```python
from build123d import *

# Parameters (mm, degrees)
F0_W      = 300
F0_H      = 160
F1_DEPTH  = 10
F2_R      = 25
F3_DEPTH  = 20.001
F4_R      = 5.5
F5_DEPTH  = 10
F6_W      = 300
F6_H      = 15
F7_DEPTH  = 20.001
F8_R      = 20
F9_R      = 27.5
F10_DEPTH = 13


with BuildPart() as f1:
    # F0 (on Front) → F1 (new body, symmetric)
    with BuildSketch(Plane.XZ):
        Rectangle(F0_W, F0_H)
    extrude(amount=F1_DEPTH, both=True)

    # F2 (on face) → F3 (cut, through all)
    with BuildSketch(Plane.XZ.offset(10)):
        with Locations((-75, 0)):
            Circle(F2_R)
        with Locations((75, 0)):
            Circle(F2_R)
    extrude(amount=-F3_DEPTH, mode=Mode.SUBTRACT)

    # F4 (on face) → F5 (cut)
    with BuildSketch(Plane.XZ.offset(10)):
        with Locations((-137.5, 0)):
            Circle(F4_R)
        with Locations((0, 50)):
            Circle(F4_R)
        with Locations((137.5, 0)):
            Circle(F4_R)
        with Locations((0, -50)):
            Circle(F4_R)
    extrude(amount=-F5_DEPTH, mode=Mode.SUBTRACT)

    # F6 (on face) → F7 (cut, through all)
    with BuildSketch(Plane.XZ.offset(10)):
        with Locations((0, -72.5)):
            Rectangle(F6_W, F6_H)
    extrude(amount=-F7_DEPTH, mode=Mode.SUBTRACT)

    # F8
    f8_edges = [f1.edges().sort_by_distance(p)[0] for p in [
        (-150, 0, 80),
        (150, 0, 80),
        (-150, 0, -65),
        (150, 0, -65),
    ]]
    fillet(f8_edges, radius=F8_R)

    # F9 (on face) → F10 (cut)
    with BuildSketch(Plane.XZ.offset(10)):
        with Locations((-75, 0)):
            Circle(F9_R)
        with Locations((75, 0)):
            Circle(F9_R)
    extrude(amount=-F10_DEPTH, mode=Mode.SUBTRACT)


solid = f1.part
```
The model under review builds one solid part; all positions refer to its coordinate system, in mm. A direction names the side the tool comes from. Round coordinates to 2 decimals unless told otherwise and drop trailing zeros. Loops run counter-clockwise (first coordinate to the right, second up) from the corner with the lowest first, then second, coordinate; pieces in that order, holes last. Notation, with made-up numbers: (33, 79) - (88, 79) arc R30 cw to (88, 102) - close; hole circle Ø4 at (-27, -18.75). An arc over 180 degrees is marked (long way). Write each question's results on one line, items separated by ' | '. Start each with the question number.
Q1. Take a section at C-C on y = 6. Give the boundary of the cut face in (x, z), plus the area to 3 significant figures.
Q2. Wall thickness on line 1 along Z through (x, y) = (0, -6.75); line 2 along X through (y, z) = (-9, -25); line 3 along Z through (x, y) = (-75, 0): over which ranges is each line inside the solid? List them lowest first. Write a range as [from, to].
Q3. Take a section at B-B on x = 75. Give the boundary of the cut face in (y, z).
Q4. Draft analysis for pull direction X (two halves, no side actions). For faces 3 (the cylindrical face through (143.986, 0.14, 74.297)), 4 (the cylindrical face through (-144.297, 0.14, -58.986)), 5 (the cylindrical face through (47.527, -3.591, 1.209)), 6 (the flat face through (-2, 0, -65)), state which applies: pulls with the +X half, pulls with the -X half, needs draft (parallel to the pull), parting line crosses it, or undercut.
Q5. Take a section at D-D on z = 50. Give the boundary of the cut face in (x, y).
Q6. Insertion check: P1, Ø5.5, axis at x = 139.5, z = 2.5, coming from the -Y side; P2, Ø10, axis at x = 0, z = 50, coming from the -Y side. Each pin has a flat end and moves straight along its axis. Give the tip position at first contact, or say it passes through.
Q7. Take a section at A-A on z = 0. Give the boundary of the cut face in (x, y), plus the area to 3 significant figures.
Q8. Tool access review of faces 1 (the cylindrical face through (-102.473, -3.591, 1.209)), 2 (the flat face through (-2, -10, 9)): name each direction out of +Z, -Z, +X, -X, +Y, -Y from which nothing blocks a thin tool from reaching the whole face with its end or side.
Data:
1) outline: (-150, -45) arc R20 ccw to (-130, -65) - (130, -65) arc R20 ccw to (150, -45) - (150, 60) arc R20 ccw to (130, 80) - (-130, 80) arc R20 ccw to (-150, 60) - close; hole circle Ø50 at (-75, 0); hole circle Ø50 at (75, 0) | area: 39,200 mm²
2) line 1: z = [-65, -55.5], [-44.5, 44.5], [55.5, 80] | line 2: x = [-150, -86.46], [-63.54, 63.54], [86.46, 150] | line 3: z = [-65, -27.5], [27.5, 80]
3) outline: (-10, -65) - (10, -65) - (10, -25) - (3, -25) - (3, -27.5) - (-10, -27.5) - close; (-10, 27.5) - (3, 27.5) - (3, 25) - (10, 25) - (10, 80) - (-10, 80) - close
4) face 3: pulls with the +X half | face 4: pulls with the -X half | face 5: undercut | face 6: needs draft
5) outline: (-150, -10) - (-5.5, -10) - (-5.5, 0) - (5.5, 0) - (5.5, -10) - (150, -10) - (150, 10) - (-150, 10) - close
6) P1: stops at y = -10 | P2: stops at y = 0
7) outline: (-150, -10) - (-143, -10) - (-143, 0) - (-132, 0) - (-132, -10) - (-102.5, -10) - (-102.5, 3) - (-100, 3) - (-100, 10) - (-150, 10) - close; (-50, 3) - (-47.5, 3) - (-47.5, -10) - (47.5, -10) - (47.5, 3) - (50, 3) - (50, 10) - (-50, 10) - close; (100, 3) - (102.5, 3) - (102.5, -10) - (132, -10) - (132, 0) - (143, 0) - (143, -10) - (150, -10) - (150, 10) - (100, 10) - close | area: 3,650 mm²
8) face 1: -Y | face 2: +Z, -Z, +X, -X, -Y
